```python
from build123d import *

# Parameters (mm, degrees)
BOSS_EXTRUDE1_DEPTH            = 50
SHELL1_START                   = 2.54
SHELL1_DEPTH                   = 47.46
SKETCH3_R                      = 45
CUT_EXTRUDE1_DEPTH             = 1.74
SKETCH4_W                      = 40
SKETCH4_H                      = 40
CUT_EXTRUDE2_DEPTH             = 1.74
F_1_0MM_DOWEL_HOLE1_AT_2_COUNT = 2
F_1_0MM_DOWEL_HOLE1_AT_2_PITCH = 99.87910309
F_1_0MM_DOWEL_HOLE1_AT_3_COUNT = 2
F_1_0MM_DOWEL_HOLE1_AT_3_PITCH = 131.082783866
F_1_0MM_DOWEL_HOLE1_AT_4_COUNT = 2
F_1_0MM_DOWEL_HOLE1_AT_4_PITCH = 131.419090104
F_1_0MM_DOWEL_HOLE1_AT_5_COUNT = 2
F_1_0MM_DOWEL_HOLE1_AT_5_PITCH = 100.320069037


# Read off the part's stored shape, not the designer's step: Shell1
with BuildPart() as part:
    # Sketch2 → Boss-Extrude1 (new body)
    with BuildSketch(Plane.XY):
        with BuildLine():
            Line((-59.862068966, 43.445816391), (-59.862068966, 43.448275862))
            Line((-59.862068966, 43.448275862), (-259.862068966, 43.448275862))
            Line((-259.862068966, 43.448275862), (-259.862068966, 163.448275862))
            Line((-259.862068966, 163.448275862), (-59.862068966, 163.448275862))
            Line((-59.862068966, 163.448275862), (-59.862068966, 163.328859089))
            ThreePointArc((-59.862068966, 163.328859089), (0.079347122, 103.38733774), (-59.862068966, 43.445816391))
        make_face()
    extrude(amount=BOSS_EXTRUDE1_DEPTH)

    # Shell1 outline → Shell1 (cut)
    with BuildSketch(Plane.XY.offset(SHELL1_START)):
        with BuildLine():
            Line((-257.322068966, 160.908275862), (-257.322068966, 45.988275862))
            Line((-257.322068966, 45.988275862), (-59.330809241, 45.988275862))
            ThreePointArc((-59.330809241, 45.988275862), (-2.481203762, 104.923202846), (-62.402068966, 160.732639099))
            Line((-62.402068966, 160.732639099), (-62.402068966, 160.908275862))
            Line((-62.402068966, 160.908275862), (-257.322068966, 160.908275862))
        make_face()
    extrude(amount=SHELL1_DEPTH, mode=Mode.SUBTRACT)

    # Sketch3 → Cut-Extrude1 (cut)
    with BuildSketch(Plane(origin=(0, 0, 0), x_dir=(-1, 0, 0), z_dir=(0, 0, -1))):
        with Locations((75.49891969, 103.730340091)):
            Circle(SKETCH3_R)
    extrude(amount=-CUT_EXTRUDE1_DEPTH, mode=Mode.SUBTRACT)

    # Sketch4 → Cut-Extrude2 (cut)
    with BuildSketch(Plane(origin=(0, 0, 0), x_dir=(-1, 0, 0), z_dir=(0, 0, -1))):
        with Locations((187.286164269, 103.448275862)):
            Rectangle(SKETCH4_W, SKETCH4_H)
    extrude(amount=-CUT_EXTRUDE2_DEPTH, mode=Mode.SUBTRACT)

    # Sketch8 → Ø1.0mm Dowel Hole1 (revolve, cut)
    with BuildSketch(Plane(origin=(-72.665980043, 104.296928021, 1.74), x_dir=(0, 1, 0), z_dir=(1, 0, 0))):
        Polygon((0, 0), (0, 1.57043031), (0.5, 1.27), (0.5, 2), (2.5, 0), align=None)
    f_1_0mm_dowel_hole1 = revolve(axis=Axis((-72.665980043, 104.296928021, -4.61), (0, 0, 1)), mode=Mode.SUBTRACT)

    # Ø1.0mm Dowel Hole1 at 2: Ø1.0mm Dowel Hole1 ×2
    with Locations(*[Vector(-0.9898926866452568, 0.1418184364821284, 0) * (i * F_1_0MM_DOWEL_HOLE1_AT_2_PITCH) for i in range(1, F_1_0MM_DOWEL_HOLE1_AT_2_COUNT)]):
        add(f_1_0mm_dowel_hole1, mode=Mode.SUBTRACT)

    # Ø1.0mm Dowel Hole1 at 3: Ø1.0mm Dowel Hole1 ×2
    with Locations(*[Vector(-0.9941444630694566, 0.10805918076841914, 0) * (i * F_1_0MM_DOWEL_HOLE1_AT_3_PITCH) for i in range(1, F_1_0MM_DOWEL_HOLE1_AT_3_COUNT)]):
        add(f_1_0mm_dowel_hole1, mode=Mode.SUBTRACT)

    # Ø1.0mm Dowel Hole1 at 4: Ø1.0mm Dowel Hole1 ×2
    with Locations(*[Vector(-0.9916004111862218, -0.12933918406776793, 0) * (i * F_1_0MM_DOWEL_HOLE1_AT_4_PITCH) for i in range(1, F_1_0MM_DOWEL_HOLE1_AT_4_COUNT)]):
        add(f_1_0mm_dowel_hole1, mode=Mode.SUBTRACT)

    # Ø1.0mm Dowel Hole1 at 5: Ø1.0mm Dowel Hole1 ×2
    with Locations(*[Vector(-0.9855415237113911, -0.16943407284436512, 0) * (i * F_1_0MM_DOWEL_HOLE1_AT_5_PITCH) for i in range(1, F_1_0MM_DOWEL_HOLE1_AT_5_COUNT)]):
        add(f_1_0mm_dowel_hole1, mode=Mode.SUBTRACT)


solid = part.part
```
Work out the finished part from the listing and answer in its coordinate system (mm). A direction names the side the tool comes from. Give positions to 0.01 mm unless a question says otherwise; leave off trailing zeros. Write each loop counter-clockwise with the first axis right and the second up, starting at its lowest first coordinate (ties: lowest second). Pieces come first, ordered by that corner, then holes. Notation, with made-up numbers: (-32, -30.75) -> (-21, -30.75) arc R16 ccw to (-21, -1.75) -> close; hole circle Ø3 at (32.25, -25.75). An arc over 180 degrees is marked (long way). Write item = value, one per line.
Q1. For a pull along X with two mould halves and no side action, classify faces 4 (the flat face through (-160, 45.988, 26)), 5 (the flat face through (-139, 162, 50)), 6 (the cylindrical face through (0.065, 104.705, 24.65)) as pulls with the +X half, pulls with the -X half, needs draft (parallel to the pull), parting line crosses it, or undercut.
Computed values:
face_4 = undercut
face_5 = needs draft
face_6 = pulls with the +X half
Q2. A tool of negligible diameter and unlimited length cuts with its end or side. For faces 1 (the flat face through (-187, 104, 1.74)), 2 (the flat face through (-259.862, 103, 25)), 3 (the flat face through (-158, 160.908, 26)), from which of +Z, -Z, +X, -X, +Y, -Y can it reach the whole face along a straight path? Write none if from no direction.
Computed values:
face_1 = -Z
face_2 = +Z, -Z, -X, +Y, -Y
face_3 = +Z
Q3. Section B-B on x = -228.5 is taken. Determine the outline of the cut face in (y, z).
Computed values:
outline = (43.45, 0) -> (163.45, 0) -> (163.45, 50) -> (160.91, 50) -> (160.91, 2.54) -> (45.99, 2.54) -> (45.99, 50) -> (43.45, 50) -> close
Q4. Section C-C on y = 68 is taken. Determine the outline of the cut face in (x, z).
Computed values:
outline = (-259.86, 0) -> (-102.85, 0) -> (-102.85, 1.74) -> (-48.14, 1.74) -> (-48.14, 0) -> (-11.48, 0) -> (-11.48, 50) -> (-14.67, 50) -> (-14.67, 2.54) -> (-257.32, 2.54) -> (-257.32, 50) -> (-259.86, 50) -> close
Q5. Consider line 1 along Y through (x, z) = (-210, 21); line 2 along Z through (x, y) = (-72.5, 123.5); line 3 along Y through (x, z) = (-18, 4.5). Determine where each line is inside the solid, lowest interval first.
Computed values:
line_1 = 43.45 to 45.99, 160.91 to 163.45
line_2 = 1.74 to 2.54
line_3 = 60.49 to 64.11, 142.66 to 146.29
Q6. Section D-D on x = -105 is taken. Determine the outline of the cut face in (y, z), and give its area (3 significant figures).
Computed values:
outline = (43.45, 0) -> (69.75, 0) -> (69.75, 1.74) -> (137.71, 1.74) -> (137.71, 0) -> (163.45, 0) -> (163.45, 50) -> (160.91, 50) -> (160.91, 2.54) -> (45.99, 2.54) -> (45.99, 50) -> (43.45, 50) -> close
area = 428 mm^2
Q7. Flat-ended cylindrical pins translate along their axes: pin 1 Ø6 at (y, z) = (109, 10) entering from +X; pin 2 Ø14 at (y, z) = (106, 36) entering from +X; pin 3 Ø1 at (x, z) = (-52, 8.5) entering from +Y (3 decimals). Find the tip coordinate at first contact, or state that the pin passes through.
Computed values:
pin_1 = 0.02
pin_2 = 0.08
pin_3 = 162.875
